from build123d import *

# Parameters (mm, degrees)
F0_W        = 40
F0_H        = 23
F1_DEPTH    = 2.4
F2_W        = 8.5
F2_H        = 23
F3_DEPTH    = 9
F4_DEPTH    = 4
F5_W        = 4.35
F5_H        = 1.8
F5_W_2      = 5.3926127389
F5_H_2      = 4.4
F6_DEPTH    = 22
F7_DEPTH    = 23.001
F8_T1_DEPTH = 22
F8_T3_DEPTH = 24.0600856157
F8_T5_DEPTH = 30.1032426749
F8_T7_DEPTH = 4
F8_T9_DEPTH = 26.5
F9_R        = 0.5
F11_DEPTH   = 4.001


# Not quite as in the source:
# - a fillet or chamfer that OpenCascade refuses, or shapes differently, is made with other operations: its cross-section is extruded or revolved along the edge and cut away or added


with BuildPart() as f1:
    # F0 (on Top) → F1 (new body)
    with BuildSketch(Plane.XY):
        Rectangle(F0_W, F0_H)
        with BuildLine():
            ThreePointArc((-11.4, 1.5), (-9.4, -0.5), (-11.4, -2.5))
            Line((-11.4, -2.5), (-13.4, -2.5))
            Line((-13.4, -2.5), (-13.4, 1.5))
            Line((-13.4, 1.5), (-11.4, 1.5))
        make_face(mode=Mode.SUBTRACT)
        with BuildLine():
            ThreePointArc((11.4, -2.5), (9.4, -0.5), (11.4, 1.5))
            Line((11.4, 1.5), (13.4, 1.5))
            Line((13.4, 1.5), (13.4, -2.5))
            Line((13.4, -2.5), (11.4, -2.5))
        make_face(mode=Mode.SUBTRACT)
        with BuildLine():
            Line((-11.4, 1.5), (-11.4, -2.5))
            ThreePointArc((-11.4, -2.5), (-9.4, -0.5), (-11.4, 1.5))
        make_face()
        with BuildLine():
            Line((11.4, -2.5), (11.4, 1.5))
            ThreePointArc((11.4, 1.5), (9.4, -0.5), (11.4, -2.5))
        make_face()
    extrude(amount=-F1_DEPTH)

    # F2 (on face) → F3 (join)
    with BuildSketch(Plane.XY):
        with Locations((15.75, 0)):
            Rectangle(F2_W, F2_H)
        with Locations((-15.75, 0)):
            Rectangle(F2_W, F2_H)
    extrude(amount=F3_DEPTH)

    # F0 (on Top) → F4 (join)
    with BuildSketch(Plane.XY):
        with BuildLine():
            Line((-11.4, 1.5), (-11.4, -2.5))
            ThreePointArc((-11.4, -2.5), (-9.4, -0.5), (-11.4, 1.5))
        make_face()
        with BuildLine():
            Line((11.4, -2.5), (11.4, 1.5))
            ThreePointArc((11.4, 1.5), (9.4, -0.5), (11.4, -2.5))
        make_face()
    extrude(amount=-F4_DEPTH)

    # F5 (on face) → F6 (cut)
    with BuildSketch(Plane(origin=(0, 11.5, 0), x_dir=(-1, 0, 0), z_dir=(0, 1, 0))):
        with Locations((-13.675, 6.7)):
            Rectangle(F5_W, F5_H)
        with Locations((13.675, 6.7)):
            Rectangle(F5_W, F5_H)
        with Locations((14.1963063695, 2.2)):
            Rectangle(F5_W_2, F5_H_2)
        with Locations((-14.1963063695, 2.2)):
            Rectangle(F5_W_2, F5_H_2)
    extrude(amount=-F6_DEPTH, mode=Mode.SUBTRACT)

    # F5 (on face) → F7 (cut, through all)
    with BuildSketch(Plane(origin=(0, 11.5, 0), x_dir=(-1, 0, 0), z_dir=(0, 1, 0))):
        Polygon((-20, 0), (-17.85, 9), (-20, 9), align=None)
        Polygon((20, 9), (17.85, 9), (20, 0), align=None)
    extrude(amount=-F7_DEPTH, mode=Mode.SUBTRACT)

    # F8: fillet of radius 1.8 on 12 edges, made by hand

    # F8_s2 → F8_t1 (join)
    with BuildSketch(Plane.XZ.offset(-11.5)):
        with BuildLine():
            ThreePointArc((15.0926127389, 0), (16.3654049451, 0.5272077939), (16.8926127389, 1.8))
            Line((16.8926127389, 1.8), (16.8926127389, 0))
            Line((16.8926127389, 0), (15.0926127389, 0))
        make_face()
        with BuildLine():
            ThreePointArc((15.0926127389, 4.4), (16.3654049451, 3.8727922061), (16.8926127389, 2.6))
            Line((16.8926127389, 2.6), (16.8926127389, 4.4))
            Line((16.8926127389, 4.4), (15.0926127389, 4.4))
        make_face()
        with BuildLine():
            ThreePointArc((-16.8926127389, 2.6), (-16.3654049451, 3.8727922061), (-15.0926127389, 4.4))
            Line((-15.0926127389, 4.4), (-16.8926127389, 4.4))
            Line((-16.8926127389, 4.4), (-16.8926127389, 2.6))
        make_face()
        with BuildLine():
            ThreePointArc((-15.0926127389, 0), (-16.3654049451, 0.5272077939), (-16.8926127389, 1.8))
            Line((-16.8926127389, 1.8), (-16.8926127389, 0))
            Line((-16.8926127389, 0), (-15.0926127389, 0))
        make_face()
    extrude(amount=F8_T1_DEPTH)

    # F8_s4 → F8_t3 (cut)
    with BuildSketch(Plane.XZ.offset(-12.0300428079)):
        with BuildLine():
            ThreePointArc((20, -0.2120171231), (19.987641981, -0.0014556176), (19.9507376137, 0.2062146401))
            Line((19.9507376137, 0.2062146401), (20, 0))
            Line((20, 0), (20, -0.2120171231))
        make_face()
        with BuildLine():
            ThreePointArc((-20, -0.2120171231), (-19.987641981, -0.0014556176), (-19.9507376137, 0.2062146401))
            Line((-19.9507376137, 0.2062146401), (-20, 0))
            Line((-20, 0), (-20, -0.2120171231))
        make_face()
    extrude(amount=F8_T3_DEPTH, mode=Mode.SUBTRACT)

    # F8_s6 → F8_t5 (cut)
    with BuildSketch(Plane.XZ.offset(-15.0516213374)):
        with BuildLine():
            ThreePointArc((18.1800890788, 7.6182317633), (17.5445157637, 8.6129432356), (16.429351465, 9))
            Line((16.429351465, 9), (17.85, 9))
            Line((17.85, 9), (18.1800890788, 7.6182317633))
        make_face()
        with BuildLine():
            ThreePointArc((-18.1800890788, 7.6182317633), (-17.5445157637, 8.6129432356), (-16.429351465, 9))
            Line((-16.429351465, 9), (-17.85, 9))
            Line((-17.85, 9), (-18.1800890788, 7.6182317633))
        make_face()
    extrude(amount=F8_T5_DEPTH, mode=Mode.SUBTRACT)

    # F8_s8 → F8_t7 (cut)
    with BuildSketch(Plane.XZ.offset(-1.5)):
        with BuildLine():
            ThreePointArc((-9.6, 0), (-10.8727922061, -0.5272077939), (-11.4, -1.8))
            Line((-11.4, -1.8), (-11.4, 0))
            Line((-11.4, 0), (-9.6, 0))
        make_face()
        with BuildLine():
            ThreePointArc((9.6, 0), (10.8727922061, -0.5272077939), (11.4, -1.8))
            Line((11.4, -1.8), (11.4, 0))
            Line((11.4, 0), (9.6, 0))
        make_face()
    extrude(amount=F8_T7_DEPTH, mode=Mode.SUBTRACT)

    # F8_s10 → F8_t9 (cut)
    with BuildSketch(Plane.XZ.offset(-16)):
        with BuildLine():
            ThreePointArc((-11.5, 6.2), (-12.0272077939, 4.9272077939), (-13.3, 4.4))
            Line((-13.3, 4.4), (-11.5, 4.4))
            Line((-11.5, 4.4), (-11.5, 6.2))
        make_face()
        with BuildLine():
            ThreePointArc((11.5, 6.2), (12.0272077939, 4.9272077939), (13.3, 4.4))
            Line((13.3, 4.4), (11.5, 4.4))
            Line((11.5, 4.4), (11.5, 6.2))
        make_face()
    extrude(amount=F8_T9_DEPTH, mode=Mode.SUBTRACT)

    # F9
    f9_edges = [f1.edges().sort_by_distance(p)[0] for p in [
        (-15.85, 11.5, 6.7),
        (-13.675, 11.5, 7.6),
        (-13.697504, 11.5, 5.8),
        (13.697504, 11.5, 5.8),
        (13.675, 11.5, 7.6),
        (15.85, 11.5, 6.7),
        (11.5, 0, 9),
        (-11.5, 0, 9),
        (0, 11.5, 0),
        (12.177503, 11.5, 4.792875),
        (14.196306, 11.5, 4.4),
        (16.365405, 11.5, 3.872792),
        (16.892613, 11.5, 2.2),
        (16.365405, 11.5, 0.527208),
        (-16.365405, 11.5, 0.527208),
        (-16.892613, 11.5, 2.2),
        (-16.365405, 11.5, 3.872792),
        (-14.196306, 11.5, 4.4),
        (-12.177503, 11.5, 4.792875),
    ]]
    fillet(f9_edges, radius=F9_R)

    # F10 (on face) → F11 (cut, through all)
    with BuildSketch(Plane.XY):
        with BuildLine():
            Line((11.5, -11.5), (11.5, -10.5))
            ThreePointArc((11.5, -10.5), (0, -7.5), (-11.5, -10.5))
            Line((-11.5, -10.5), (-11.5, -11.5))
            Line((-11.5, -11.5), (11.5, -11.5))
        make_face()
    extrude(amount=-F11_DEPTH, mode=Mode.SUBTRACT)


solid = f1.part
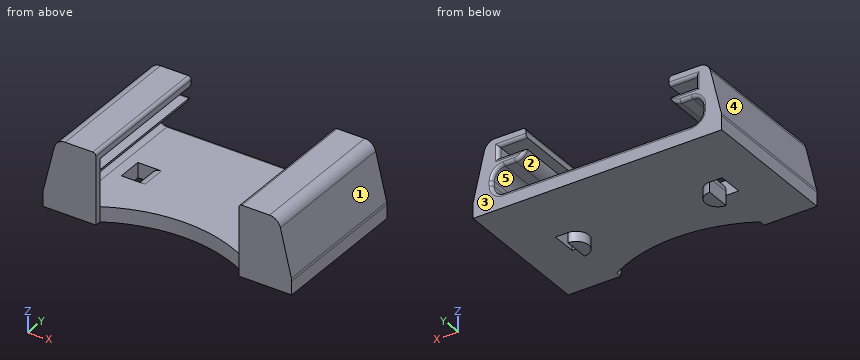
Check sheet for the modelled part. Datum: model origin and axes. Units: mm. Face numbers are marked on the shaded views. A direction names the side the tool comes from. Give positions to 0.01 mm unless a question says otherwise; leave off trailing zeros. Write each loop counter-clockwise with the first axis right and the second up, starting at its lowest first coordinate (ties: lowest second). Pieces come first, ordered by that corner, then holes. Notation, with made-up numbers: (-7, 38) -> (4, 38) arc R25 ccw to (4, 55) -> close; hole circle Ø8 at (2.25, 78.5). An arc over 180 degrees is marked (long way). Write item = value, one per line.
Item 1: Release check for a two-part mould opening along Z. For the marked faces 1, 2 and 3 record: +Z half, -Z half, draft (parallel to the pull), parting line (faces both ways), or undercut.
Output:
face_1 = +Z half
face_2 = undercut
face_3 = draft
Item 2: Sectioned sample at C-C on y = -0.5. Count the separate pieces of the cut face and the enclosed holes in it, and give its area (3 significant figures).
Output:
separate_pieces = 3
enclosed_holes = 0
area = 162 mm^2
Item 3: Scan lines: probe 1 along Z at (x, y) = (-14.5, -0.5); probe 2 along X at (y, z) = (-1.75, -2.25); probe 3 along X at (y, z) = (6, 3). Record each from-to range of solid material in increasing order. Write a range as from..to.
Output:
probe_1 = -2.4..0, 4.4..5.8, 7.6..9
probe_2 = -20..-13.4, -11.4..11.4, 13.4..20
probe_3 = -19.28..-16.85, 16.85..19.28
Item 4: Sectioned sample at B-B on x = -2.5. Record the boundary of the cut face in (y, z).
Output:
outline = (-7.63, -2.4) -> (11.5, -2.4) -> (11.5, -0.5) arc R0.5 ccw to (11, 0) -> (-7.63, 0) -> close
Item 5: Gauge pin test, flat ends, axial feed: pin 1 (0.7 mm diameter, centred on x = 10.5, z = -0.5, fed in from -Y); pin 2 (0.9 mm diameter, centred on y = -0.5, z = 6.5, fed in from -X); pin 3 (2 mm diameter, centred on x = 8.5, y = -2, fed in from -Z). Record the tip position at first contact, or that the pin passes through.
Output:
pin_1 = -10.15
pin_2 = -18.55
pin_3 = -2.4
Item 6: Tool access check on the marked faces 4 and 5. Record the directions out of +Z, -Z, +X, -X, +Y, -Y that give a thin tool (end or side, any length) a straight path to the whole face; none if there is none.
Output:
face_4 = +Z, -X, +Y, -Y
face_5 = +Y
